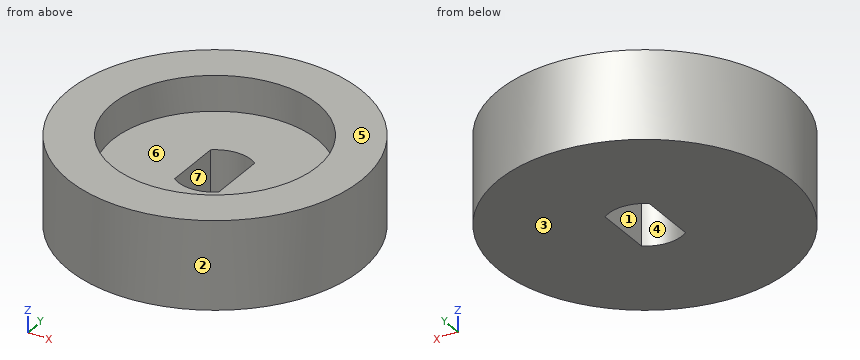
```python
from build123d import *

# Parameters (mm, degrees)
SKETCH1_R           = 10
BOSS_EXTRUDE1_DEPTH = 3
SKETCH2_R           = 7
CUT_EXTRUDE1_DEPTH  = 2.4


with BuildPart() as part:
    # Sketch1 → Boss-Extrude1 (new, symmetric)
    with BuildSketch(Plane.XY):
        Circle(SKETCH1_R)
        with BuildLine():
            Line((-1.521572539, 1.983637318), (-1.521572539, -2.016362682))
            ThreePointArc((-1.521572539, -2.016362682), (-0.016245384, -2.500087973), (1.478251514, -1.983871914))
            Line((1.478251514, -1.983871914), (1.478251514, 2.016128086))
            ThreePointArc((1.478251514, 2.016128086), (-0.02707564, 2.499853378), (-1.521572539, 1.983637318))
        make_face(mode=Mode.SUBTRACT)
    extrude(amount=BOSS_EXTRUDE1_DEPTH, both=True)

    # Sketch2 → Cut-Extrude1 (cut)
    with BuildSketch(Plane.XY.offset(3)):
        Circle(SKETCH2_R)
    extrude(amount=-CUT_EXTRUDE1_DEPTH, mode=Mode.SUBTRACT)


solid = part.part
```
Can you work these out from the model? Positions are in its coordinate system, mm. Face numbers are marked on the shaded views. A direction names the side the tool comes from. Coordinates: 2 decimals unless noted, no trailing zeros. Write each loop counter-clockwise with the first axis right and the second up, starting at its lowest first coordinate (ties: lowest second). Pieces come first, ordered by that corner, then holes. Notation, with made-up numbers: (-14.75, -0.75) - (9.25, -0.75) arc R18 cw to (9.25, 20.25) - close; hole circle Ø11 at (72.5, 41.25). An arc over 180 degrees is marked (long way). Return JSON: item names as keys, results as strings.
Q1. If we section it at B-B (x = -0.75): Please give me the cut outline in (y, z).
Computed values:
{"outline": "(-9.97, -3) - (-2.4, -3) - (-2.4, 0.6) - (-6.96, 0.6) - (-6.96, 3) - (-9.97, 3) - close; (2.38, -3) - (9.97, -3) - (9.97, 3) - (6.96, 3) - (6.96, 0.6) - (2.38, 0.6) - close"}
Q2. If we section it at D-D (x = 5.75): Please give me the cut outline in (y, z), then the cut area to 3 significant figures.
Computed values:
{"outline": "(-8.18, -3) - (8.18, -3) - (8.18, 3) - (3.99, 3) - (3.99, 0.6) - (-3.99, 0.6) - (-3.99, 3) - (-8.18, 3) - close", "area": "79.0 mm2"}
Q3. Thinking about a two-plate mould opening in Y: for the marked faces 1, 2, 3 and 4, which applies, +Y half, -Y half, draft (parallel to the pull), parting line (faces both ways), or undercut?
Computed values:
{"face 1": "undercut", "face 2": "parting line", "face 3": "draft", "face 4": "undercut"}
Q4. On a 3-axis mill with a long thin cutter (end or side, diameter ignored), from which of +Z, -Z, +X, -X, +Y, -Y can I reach the whole of each face in a straight line? I mean the marked faces 5, 6 and 7. Say none if no direction works.
Computed values:
{"face 5": "+Z, +X, -X, +Y, -Y", "face 6": "+Z", "face 7": "+Z, -Z"}
Q5. If we section it at C-C (z = -0.1): Please give me the cut outline in (x, y), then the cut area to 3 significant figures.
Computed values:
{"outline": "circle Ø20 at (0, 0); hole (-1.52, -2.02) arc R2.5 ccw to (1.48, -1.98) - (1.48, 2.02) arc R2.5 ccw to (-1.52, 1.98) - close", "area": "300 mm2"}
Q6. Please list where these lines run through material, in increasing order: L1, parallel to Y at x = 0, z = 1.7; L2, parallel to Z at x = 4.25, y = -2; L3, parallel to X at y = -5.25, z = 2.1. Write a range as from..to.
Computed values:
{"L1": "y = -10..-7, 7..10", "L2": "z = -3..0.6", "L3": "x = -8.51..-4.63, 4.63..8.51"}
Q7. If we section it at A-A (y = 0): Please give me the cut outline in (x, z).
Computed values:
{"outline": "(-10, -3) - (-1.52, -3) - (-1.52, 0.6) - (-7, 0.6) - (-7, 3) - (-10, 3) - close; (1.48, -3) - (10, -3) - (10, 3) - (7, 3) - (7, 0.6) - (1.48, 0.6) - close"}
Q8. I'm going to push flat-ended pins straight in: pin 1 Ø3 at (y, z) = (-2.5, -1.5) entering from -X; pin 2 Ø1 at (y, z) = (7, -2) entering from -X; pin 3 Ø3 at (y, z) = (2, 1.5) entering from +X. Where does each tip first touch, or does it pass through?
Computed values:
{"pin 1": "stops at x = -9.95", "pin 2": "stops at x = -7.6", "pin 3": "stops at x = 9.99"}
